Can you work these out from the drawing? Everything is in mm from the part's minimum corner. A direction names the side the tool comes from. Give positions to 0.01 mm unless a question says otherwise; leave off trailing zeros. Order: outer loops, then holes, each group sorted by start corner. A loop starts at its lowest first (then second) coordinate and runs counter-clockwise, first axis right, second up. Notation, with made-up numbers: (22.25, 6.5) - (47.25, 6.5) arc R28 ccw to (47.25, 38.5) - close; hole circle Ø9 at (7.5, 32.25). An arc over 180 degrees is marked (long way). Answer as a JSON object with one key per item and string values.
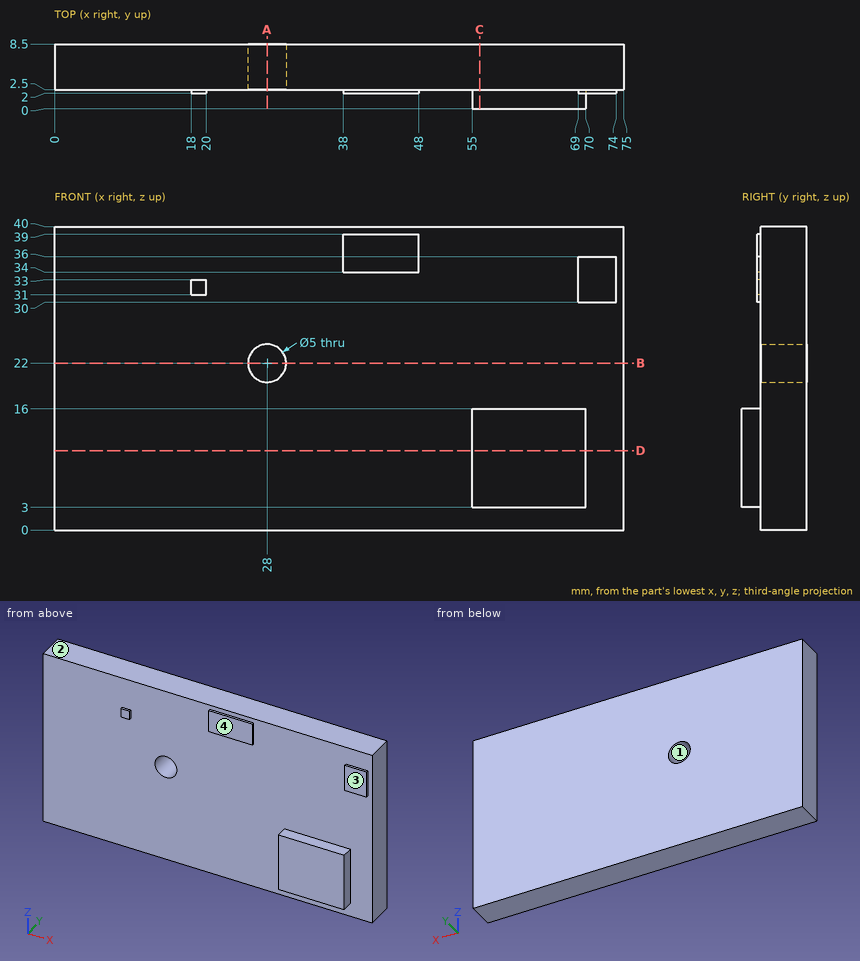
Q1. I'm going to push flat-ended pins straight in: pin 1 Ø5.5 at (x, z) = (72.5, 32.5) entering from -Y; pin 2 Ø8 at (x, z) = (47, 27.5) entering from -Y; pin 3 Ø0.8 at (x, y) = (63.5, 1) entering from +Z. Where does each tip first touch, or does it pass through?
Recorded:
{"pin 1": "stops at y = 2", "pin 2": "stops at y = 2.5", "pin 3": "stops at z = 16"}
Q2. Which directions (+Z, -Z, +X, -X, +Y, -Y) give clear straight access to the entire face, cutting with the end or side of a thin tool? Please do the marked faces 3 and 4.
Recorded:
{"face 3": "+Z, +X, -X, -Y", "face 4": "+Z, -Z, +X, -X, -Y"}
Q3. If we section it at D-D, the plane z = 10.5: Please give me the cut outline in (x, y).
Recorded:
{"outline": "(0, 2.5) - (55, 2.5) - (55, 0) - (70, 0) - (70, 2.5) - (75, 2.5) - (75, 8.5) - (0, 8.5) - close"}
Q4. If we section it at A-A, the plane x = 28: Please give me the cut outline in (y, z).
Recorded:
{"outline": "(2.5, 0) - (8.5, 0) - (8.5, 19.5) - (2.5, 19.5) - close; (2.5, 24.5) - (8.5, 24.5) - (8.5, 40) - (2.5, 40) - close"}
Q5. We'd pull the mould along X, two halves only. Please class the marked faces 1 and 2: released by +X, released by -X, zero draft, split by the parting line, or undercut.
Recorded:
{"face 1": "undercut", "face 2": "zero draft"}
Q6. I need wall thicknesses on L1, parallel to Z at x = 28, y = 5.3; L2, parallel to Y at x = 33, z = 26; L3, parallel to Z at x = 65, y = 1.75. Which ranges of each line are inside material? Lowest first, please.
Recorded:
{"L1": "z = 0 to 19.5, 24.5 to 40", "L2": "y = 2.5 to 8.5", "L3": "z = 3 to 16"}
Q7. If we section it at C-C, the plane x = 56: Please give me the cut outline in (y, z).
Recorded:
{"outline": "(0, 3) - (2.5, 3) - (2.5, 0) - (8.5, 0) - (8.5, 40) - (2.5, 40) - (2.5, 16) - (0, 16) - close"}
Q8. If we section it at B-B, the plane z = 22: Please give me the cut outline in (x, y), then the cut area to 3 significant figures.
Recorded:
{"outline": "(0, 2.5) - (25.5, 2.5) - (25.5, 8.5) - (0, 8.5) - close; (30.5, 2.5) - (75, 2.5) - (75, 8.5) - (30.5, 8.5) - close", "area": "420 mm^2"}
